```python
from build123d import *

# Parameters (mm, degrees)
BOSS_EXTRUDE1_DEPTH = 20
BOSS_EXTRUDE2_DEPTH = 5
SKETCH3_W           = 3.175
SKETCH3_H           = 13
CUT_EXTRUDE1_DEPTH  = 3


with BuildPart() as part:
    # Sketch1 → Boss-Extrude1 (new body)
    with BuildSketch(Plane(origin=(0, 0, 0), x_dir=(0, 0, -1), z_dir=(1, 0, 0))):
        Polygon((0, 0), (3, 0), (3, 10), (6.175, 10), (6.175, -22.812), (9.175, -22.812), (9.175, 15), (0, 15), align=None)
    extrude(amount=BOSS_EXTRUDE1_DEPTH)

    # Sketch2 → Boss-Extrude2 (add)
    with BuildSketch(Plane(origin=(0, 0, -9.175), x_dir=(-1, 0, 0), z_dir=(0, 0, -1))):
        Polygon((-11.5875, -22.812), (-11.5875, -9.812), (-8.4125, -9.812), (-8.4125, -22.812), (-5.4125, -22.812), (-5.4125, -6.812), (-14.5875, -6.812), (-14.5875, -22.812), align=None)
    extrude(amount=BOSS_EXTRUDE2_DEPTH)

    # Sketch3 → Cut-Extrude1 (cut)
    with BuildSketch(Plane(origin=(0, 0, -9.175), x_dir=(-1, 0, 0), z_dir=(0, 0, -1))):
        with Locations((-10, -16.312)):
            Rectangle(SKETCH3_W, SKETCH3_H)
    extrude(amount=-CUT_EXTRUDE1_DEPTH, mode=Mode.SUBTRACT)


solid = part.part
```
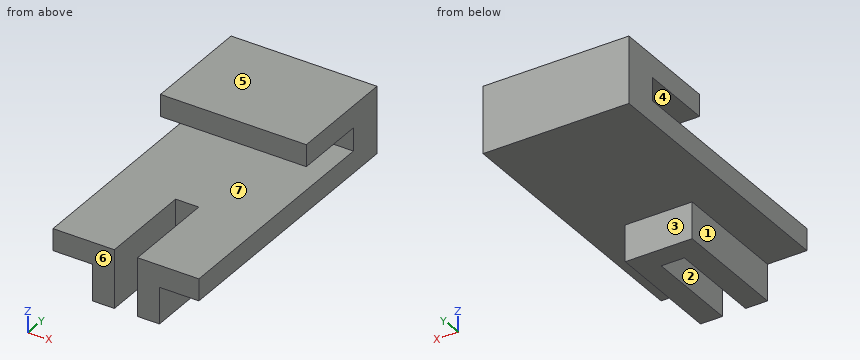
Geometry check sheet. Reference: the model listing, model coordinates, mm. Face numbers are marked on the shaded views. A direction names the side the tool comes from. Coordinates: 2 decimals unless noted, no trailing zeros. Write each loop counter-clockwise with the first axis right and the second up, starting at its lowest first coordinate (ties: lowest second). Pieces come first, ordered by that corner, then holes. Notation, with made-up numbers: (60.5, -36.5) -> (67.5, -36.5) arc R11 cw to (67.5, -21.5) -> close; hole circle Ø1 at (63.5, -7.75). An arc over 180 degrees is marked (long way). Use CSV: the item, a comma, the result in double quotes. Start each with the question number.
Item 1: Cross-section at B-B, the plane x = 2.75. Record the cut outline in (y, z) (3 decimals), plus the area to 3 significant figures.
Item 2: Set-up check for the marked faces 1, 2, 3 and 4: record each of +Z, -Z, +X, -X, +Y, -Y from which the full face is reachable in a straight line by a thin tool's end or side.
Item 3: Depth check by flat-ended pin: pin 1 Ø6 at (x, y) = (7.5, -12.5) entering from +Z (3 decimals); pin 2 Ø1 at (x, y) = (7.5, -4.5) entering from -Z (3 decimals); pin 3 Ø4 at (y, z) = (-6, -12.5) entering from -X. Enter the tip coordinate at first touch or a pass-through.
Item 4: Mould release check, pull along Z, two halves, no side actions. Record for the marked faces 5, 6 and 7: released by +Z, released by -Z, zero draft, split by the parting line, or undercut.
Item 5: Cross-section at D-D, the plane y = 1.5. Record the cut outline in (x, z) (3 decimals), plus the area to 3 significant figures.
Item 6: Cross-section at C-C, the plane z = -12. Record the cut outline in (x, y), plus the area to 3 significant figures.
Item 7: Cross-section at A-A, the plane y = -12.5. Record the cut outline in (x, z) (1 decimal), plus the area to 3 significant figures.
Item 8: Thickness scan on line 1 (Z direction, x = 8.75, y = 7) (3 decimals); line 2 (X direction, y = -13, z = -9.5); line 3 (X direction, y = -16, z = -7). Record the ranges inside material, lowest first.
Answers:
1,outline,"(-22.812, -9.175) -> (15, -9.175) -> (15, 0) -> (0, 0) -> (0, -3) -> (10, -3) -> (10, -6.175) -> (-22.812, -6.175) -> close"
1,area,"174 mm^2"
2,face 1,"-Z, -X, +Y, -Y"
2,face 2,"+Z, -Z, -Y"
2,face 3,"-Z, +X, -X, +Y"
2,face 4,"+X, -X, -Y"
3,pin 1,"z = -6.175"
3,pin 2,"z = -9.175"
3,pin 3,"x = 5.41"
4,face 5,"released by +Z"
4,face 6,"zero draft"
4,face 7,"undercut"
5,outline,"(0, -9.175) -> (20, -9.175) -> (20, -6.175) -> (0, -6.175) -> close; (0, -3) -> (20, -3) -> (20, 0) -> (0, 0) -> close"
5,area,"120 mm^2"
6,outline,"(5.41, -22.81) -> (8.41, -22.81) -> (8.41, -9.81) -> (11.59, -9.81) -> (11.59, -22.81) -> (14.59, -22.81) -> (14.59, -6.81) -> (5.41, -6.81) -> close"
6,area,"106 mm^2"
7,outline,"(0, -9.2) -> (5.4, -9.2) -> (5.4, -14.2) -> (8.4, -14.2) -> (8.4, -6.2) -> (0, -6.2) -> close; (11.6, -14.2) -> (14.6, -14.2) -> (14.6, -9.2) -> (20, -9.2) -> (20, -6.2) -> (11.6, -6.2) -> close"
7,area,"80.5 mm^2"
8,line 1,"-9.175 to -6.175, -3 to 0"
8,line 2,"5.41 to 8.41, 11.59 to 14.59"
8,line 3,"0 to 8.41, 11.59 to 20"
